Solid Edge part; units mm, degrees
sketch "Sketch1" plane through (0, 0, 0) normal (0, -1, 0) x (1, 0, 0)
  line L0 (-15, -15) -> (15, -15)
  line L1 (15, -15) -> (15, -9)
  line L2 (10, -4) -> (15, -9)
  line L3 (10, 4) -> (10, -4)
  line L4 (15, 9) -> (10, 4)
  line L5 (15, 9) -> (15, 15)
  line L6 (15, 15) -> (-15, 15)
  line L7 (-15, 15) -> (-15, 9)
  line L8 (-10, 4) -> (-15, 9)
  line L9 (-10, 4) -> (-10, -4)
  line L10 (-10, -4) -> (-15, -9)
  line L11 (-15, -9) -> (-15, -15)
  dimension "D1" = 10
extrude "Protrusion1" add sketch "Sketch1" against normal blind 300
Input: part model. Units: mm. Frame: model coordinates. A direction names the side the tool comes from. Give positions to 0.01 mm unless a question says otherwise; leave off trailing zeros. Loops run counter-clockwise (first coordinate to the right, second up) from the corner with the lowest first, then second, coordinate; pieces in that order, holes last. Notation, with made-up numbers: M 37,-7 L 49,-7 A15 ccw 49,8 Z; hole C 6,66.5 d9. An arc over 180 degrees is marked long. Use one line per item in the form item = value.
1. Line query: L1, parallel to Z at x = -13.5, y = 82; L2, parallel to Z at x = -10.25, y = 122; L3, parallel to X at y = 190, z = -2.75. Output: solid intervals per line, ascending.
Numbers:
L1 = -15 to -7.5, 7.5 to 15
L2 = -15 to -4.25, 4.25 to 15
L3 = -10 to 10
2. First-contact query: pin 1 (6 mm diameter, centred on y = 80.5, z = 5, fed in from -X); pin 2 (3 mm diameter, centred on x = -12, z = 0, fed in from +Y); pin 3 (4 mm diameter, centred on y = 219.5, z = -1.5, fed in from -X); pin 4 (6.5 mm diameter, centred on y = 76, z = 1.5, fed in from +X). Flat tips, straight axial feed; report the tip coordinate or a pass-through.
Numbers:
pin_1 = -14
pin_2 = through
pin_3 = -10
pin_4 = 10.75
3. Pull-direction query (Z, two-part tool) for faces 1 (the face through (-12, 148, 6)), 2 (the face through (0, 148, 15)), 3 (the face through (15, 148, -12)); classes: released by +Z, released by -Z, zero draft, split by the parting line, or undercut.
Numbers:
face_1 = undercut
face_2 = released by +Z
face_3 = zero draft
4. Reachability of faces 4 (the face through (-12, 148, -6)), 5 (the face through (0, 300, 0)), 6 (the face through (13, 148, 7)) from +Z, -Z, +X, -X, +Y, -Y: full face, straight path, thin tool, end or side. Return the list, or none.
Numbers:
face_4 = -X, +Y, -Y
face_5 = +Z, -Z, +X, -X, +Y
face_6 = +X, +Y, -Y
5. Section query A-A, the plane y = 74.5. Return the cut outline in (x, z), and give its area (3 significant figures).
Numbers:
outline = M -15,-15 L 15,-15 L 15,-9 L 10,-4 L 10,4 L 15,9 L 15,15 L -15,15 L -15,9 L -10,4 L -10,-4 L -15,-9 Z
area = 770 mm²
6. Section query B-B, the plane z = 1.5. Return the cut outline in (x, y), and give its area (3 significant figures).
Numbers:
outline = M -10,0 L 10,0 L 10,300 L -10,300 Z
area = 6,000 mm²
